```python
from build123d import *

# Parameters (mm, degrees)
BOSS_EXTRUDE1_DEPTH = 30
SKETCH2_R           = 2
CUT_EXTRUDE1_DEPTH  = 7
FILLET1_R           = 10
FILLET2_R           = 5


with BuildPart() as part:
    # Sketch1 → Boss-Extrude1 (new body)
    with BuildSketch(Plane(origin=(0, 0, 0), x_dir=(1, 0, 0), z_dir=(0, 1, 0))):
        with BuildLine():
            ThreePointArc((-24.171263931, 4), (0, 24.5), (24.171263931, 4))
            Line((24.171263931, 4), (49.171263931, 4))
            Line((49.171263931, 4), (49.171263931, 10))
            Line((49.171263931, 10), (30.397368307, 10))
            ThreePointArc((30.397368307, 10), (0, 32), (-30.397368307, 10))
            Line((-30.397368307, 10), (-49.171263931, 10))
            Line((-49.171263931, 10), (-49.171263931, 4))
            Line((-49.171263931, 4), (-24.171263931, 4))
        make_face()
    extrude(amount=BOSS_EXTRUDE1_DEPTH)

    # Sketch2 → Cut-Extrude1 (cut, through all)
    with BuildSketch(Plane(origin=(0, 0, -10), x_dir=(-1, 0, 0), z_dir=(0, 0, -1))):
        with Locations((-39.171263931, 22)):
            Circle(SKETCH2_R)
        with Locations((-39.171263931, 8)):
            Circle(SKETCH2_R)
        with Locations((39.171263931, 8)):
            Circle(SKETCH2_R)
        with Locations((39.171263931, 22)):
            Circle(SKETCH2_R)
    extrude(amount=-CUT_EXTRUDE1_DEPTH, mode=Mode.SUBTRACT)

    # Fillet1
    fillet1_edges = [part.edges().sort_by_distance(p)[0] for p in [
        (-30.397368307, 15, -10),
        (30.397368307, 15, -10),
    ]]
    fillet(fillet1_edges, radius=FILLET1_R)

    # Fillet2
    fillet2_edges = [part.edges().sort_by_distance(p)[0] for p in [
        (-24.171263931, 15, -4),
        (24.171263931, 15, -4),
    ]]
    fillet(fillet2_edges, radius=FILLET2_R)


solid = part.part
```
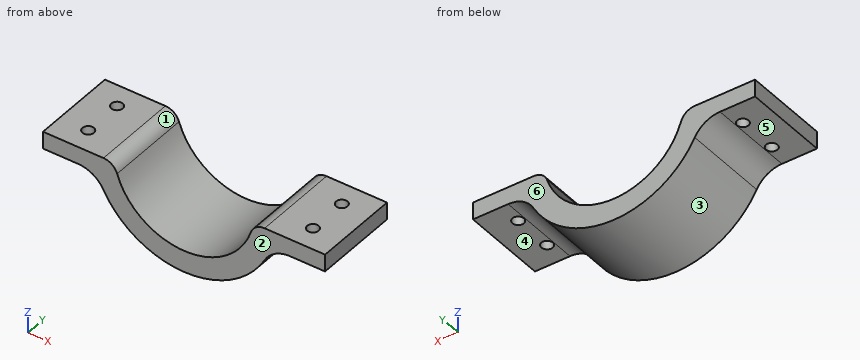
The model under review builds one solid part; all positions refer to its coordinate system, in mm. Face numbers are marked on the shaded views. A direction names the side the tool comes from. Round coordinates to 2 decimals unless told otherwise and drop trailing zeros. Loops run counter-clockwise (first coordinate to the right, second up) from the corner with the lowest first, then second, coordinate; pieces in that order, holes last. Notation, with made-up numbers: M -12,-34 L 43,-34 A24 ccw 43,-18 Z; hole C 13.5,70 d11. An arc over 180 degrees is marked long. Answer as a JSON object with one key per item and string values.
(1) Take a section at B-B on y = 8. Give the boundary of the cut face in (x, z).
Resolved:
{"outline": "M -49.17,-10 L -41.17,-10 L -41.17,-4 L -49.17,-4 Z; M -37.17,-10 L -36.93,-10 A10 cw -28.14,-15.24 A32 ccw 28.14,-15.24 A10 cw 36.93,-10 L 37.17,-10 L 37.17,-4 L 28.09,-4 A5 ccw 23.33,-7.47 A24.5 cw -23.33,-7.47 A5 ccw -28.09,-4 L -37.17,-4 Z; M 41.17,-10 L 49.17,-10 L 49.17,-4 L 41.17,-4 Z"}
(2) Tool access review of the marked faces 4, 5 and 6: name each direction out of +Z, -Z, +X, -X, +Y, -Y from which nothing blocks a thin tool from reaching the whole face with its end or side.
Resolved:
{"face 4": "-Z, +X, +Y, -Y", "face 5": "-Z, -X, +Y, -Y", "face 6": "+Z, -Z, +X, -X, +Y"}
(3) Draft analysis for pull direction X (two halves, no side actions). For the marked faces 1, 2 and 3, state which applies: released by +X, released by -X, zero draft, split by the parting line, or undercut.
Resolved:
{"face 1": "undercut", "face 2": "zero draft", "face 3": "split by the parting line"}
(4) Take a section at C-C on y = 15.25. Give the boundary of the cut face in (x, z), and give its area (3 significant figures).
Resolved:
{"outline": "M -49.17,-10 L -36.93,-10 A10 cw -28.14,-15.24 A32 ccw 28.14,-15.24 A10 cw 36.93,-10 L 49.17,-10 L 49.17,-4 L 28.09,-4 A5 ccw 23.33,-7.47 A24.5 cw -23.33,-7.47 A5 ccw -28.09,-4 L -49.17,-4 Z", "area": "830 mm²"}
(5) Clearance check with flat-ended pins moving along their axes: P1, Ø12, axis at x = -34.5, y = 27, coming from the -Z side; P2, Ø12, axis at y = 5.5, z = -18.5, coming from the -X side; P3, Ø6, axis at y = 24, z = -24.5, coming from the -X side; P4, Ø6, axis at x = -12, z = -18, coming from the +Y side. State where each tip first meets the part, or that it passes through.
Resolved:
{"P1": "z = -14.62", "P2": "x = -30.32", "P3": "x = -23.7", "P4": "y = 30"}
(6) Take a section at D-D on z = -13.5. Give the boundary of the cut face in (x, y).
Resolved:
{"outline": "M -29.33,0 L -20.45,0 L -20.45,30 L -29.33,30 Z; M 20.45,0 L 29.33,0 L 29.33,30 L 20.45,30 Z"}
(7) Take a section at A-A on z = -22.25. Give the boundary of the cut face in (x, y), and give its area (3 significant figures).
Resolved:
{"outline": "M -23,0 L -10.26,0 L -10.26,30 L -23,30 Z; M 10.26,0 L 23,0 L 23,30 L 10.26,30 Z", "area": "765 mm²"}
(8) To check wall thickness, follow line 1 along Z through (x, y) = (-42.5, 12); line 2 along X through (y, z) = (18, -9.75); line 3 along X through (y, z) = (12.25, -15.5). State the ranges of each line that lie inside material, in increasing order.
Resolved:
{"line 1": "-10 to -4", "line 2": "-49.17 to -22.48, 22.48 to 49.17", "line 3": "-28 to -18.97, 18.97 to 28"}
